from build123d import *

# Parameters (mm, degrees)
CROQUIS1_R              = 12
CROQUIS1_R_2            = 3.25
SALIENTE_EXTRUIR1_DEPTH = 35
SALIENTE_EXTRUIR2_START = -10
CROQUIS2_R              = 12
CROQUIS2_R_2            = 8
SALIENTE_EXTRUIR2_DEPTH = 10
CROQUIS3_R              = 5.1
CROQUIS3_W              = 8
CROQUIS3_H              = 16.86
CORTAR_EXTRUIR2_DEPTH   = 105.669140151


with BuildPart() as part:
    # Croquis1 → Saliente-Extruir1 (new body)
    # profile 1 of 2: a face of its own
    with BuildSketch(Plane.XY):
        with BuildLine():
            Line((0, 85.17), (0, 40.17))
            Line((0, 40.17), (10, 40.17))
            Line((10, 40.17), (10, 60.17))
            Line((10, 60.17), (30, 60.17))
            Line((30, 60.17), (30, 40.17))
            Line((30, 40.17), (40, 40.17))
            Line((40, 40.17), (40, 85.17))
            ThreePointArc((40, 85.17), (38.535533906, 88.705533906), (35, 90.17))
            Line((35, 90.17), (5, 90.17))
            ThreePointArc((5, 90.17), (1.464466094, 88.705533906), (0, 85.17))
        make_face()
        with Locations((20, 74.17)):
            Circle(CROQUIS1_R, mode=Mode.SUBTRACT)
    # profile 2 of 2: a face of its own
    with BuildSketch(Plane.XY):
        with BuildLine():
            Line((5, 0), (35, 0))
            ThreePointArc((35, 0), (38.535533906, 1.464466094), (40, 5))
            Line((40, 5), (40, 40.17))
            Line((40, 40.17), (0, 40.17))
            Line((0, 40.17), (0, 5))
            ThreePointArc((0, 5), (1.464466094, 1.464466094), (5, 0))
        make_face()
        with Locations((20, 4)):
            Circle(CROQUIS1_R_2, mode=Mode.SUBTRACT)
    extrude(amount=SALIENTE_EXTRUIR1_DEPTH)

    # Croquis2 → Saliente-Extruir2 (add)
    with BuildSketch(Plane.XY.offset(35).offset(SALIENTE_EXTRUIR2_START)):
        with Locations((20, 74.17)):
            Circle(CROQUIS2_R)
        with Locations((20, 74.17)):
            Circle(CROQUIS2_R_2, mode=Mode.SUBTRACT)
    extrude(amount=SALIENTE_EXTRUIR2_DEPTH)

    # Croquis3 → Cortar-Extruir2 (cut, through all)
    with BuildSketch(Plane.ZY):
        with Locations((17.5, 27.36)):
            Circle(CROQUIS3_R)
        with Locations((17.5, 8.43)):
            Rectangle(CROQUIS3_W, CROQUIS3_H)
    extrude(amount=-CORTAR_EXTRUIR2_DEPTH, mode=Mode.SUBTRACT)


solid = part.part
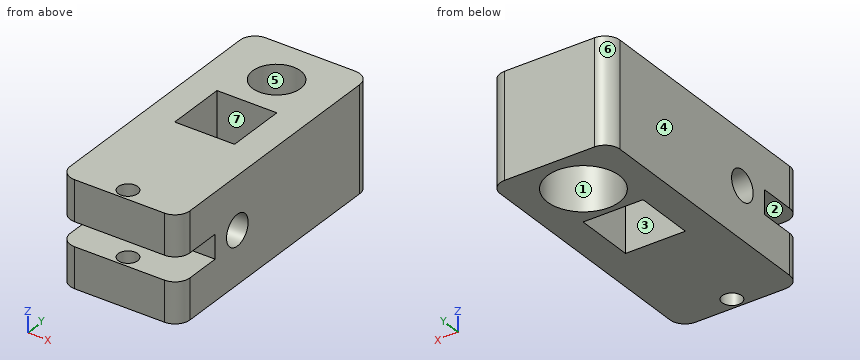
The listing builds one solid part. Answer for the finished solid, in the listing's coordinates (mm). Face numbers are marked on the shaded views. A direction names the side the tool comes from. Coordinates: 2 decimals unless noted, no trailing zeros. Loops run counter-clockwise (first coordinate to the right, second up) from the corner with the lowest first, then second, coordinate; pieces in that order, holes last. Notation, with made-up numbers: (76, 25.5) -> (117, 25.5) arc R29 cw to (117, 58.5) -> close; hole circle Ø9 at (20, 11.25). An arc over 180 degrees is marked (long way). Answer in a Markdown table with one row per item. Add a question column.
1. The part is cut by section C-C, the plane y = 27.36. Write down the section's boundary in (x, z), then the cut area to 3 significant figures.
2. The part is cut by section D-D, the plane z = 31.5. Write down the section's boundary in (x, y), then the cut area to 3 significant figures.
3. The part is cut by section A-A, the plane x = 20. Count the separate pieces of the cut face and the enclosed holes in it, then the cut area to 3 significant figures.
4. Flat-ended cylindrical pins translate along their axes: P1, Ø1.5, axis at x = 27, z = 20, coming from the -Y side; P2, Ø21, axis at x = 20, y = 74.17, coming from the -Z side; P3, Ø4, axis at x = 20, y = 4, coming from the +Z side. Find the tip coordinate at first contact, or state that the pin passes through.
5. For the marked faces 1, 2 and 3, determine the directions among +Z, -Z, +X, -X, +Y, -Y from which every point of the face is accessible in a straight line to the end or side of a thin tool.
6. Consider line 1 (Y direction, x = 20, z = 29); line 2 (X direction, y = 52, z = 9); line 3 (Z direction, x = 30, y = 27). Determine where each line is inside the solid, lowest interval first. Write a range as [from, to].
7. The part is cut by section B-B, the plane z = 17.5. Write down the section's boundary in (x, y), then the cut area to 3 significant figures.
8. Determine the mould class of the marked faces 4, 5, 6 and 7 for opening direction Y: +Y half, -Y half, draft (parallel to the pull), parting line (faces both ways), or undercut.
Answer below:
| question | item | result |
|---|---|---|
| 1 | outline | (0, 0) -> (40, 0) -> (40, 12.4) -> (0, 12.4) -> close; (0, 22.6) -> (40, 22.6) -> (40, 35) -> (0, 35) -> close |
| 1 | area | 992 mm2 |
| 2 | outline | (0, 5) arc R5 ccw to (5, 0) -> (35, 0) arc R5 ccw to (40, 5) -> (40, 85.17) arc R5 ccw to (35, 90.17) -> (5, 90.17) arc R5 ccw to (0, 85.17) -> close; hole (10, 40.17) -> (30, 40.17) -> (30, 60.17) -> (10, 60.17) -> close; hole circle Ø16 at (20, 74.17); hole circle Ø6.5 at (20, 4) |
| 2 | area | 2,950 mm2 |
| 3 | separate pieces | 5 |
| 3 | enclosed holes | 1 |
| 3 | area | 1,300 mm2 |
| 4 | P1 | y = 16.86 |
| 4 | P2 | z = 25 |
| 4 | P3 | through |
| 5 | face 1 | -Z |
| 5 | face 2 | +X, -X, -Y |
| 5 | face 3 | +Z, -Z |
| 6 | line 1 | [0, 0.75], [7.25, 40.17], [60.17, 66.17], [82.17, 90.17] |
| 6 | line 2 | [0, 10], [30, 40] |
| 6 | line 3 | [0, 12.41], [22.59, 35] |
| 7 | outline | (0, 16.86) -> (40, 16.86) -> (40, 22.26) -> (0, 22.26) -> close; (0, 32.46) -> (40, 32.46) -> (40, 85.17) arc R5 ccw to (35, 90.17) -> (5, 90.17) arc R5 ccw to (0, 85.17) -> close; hole circle Ø24 at (20, 74.17); hole (10, 40.17) -> (30, 40.17) -> (30, 60.17) -> (10, 60.17) -> close |
| 7 | area | 1,660 mm2 |
| 8 | face 4 | draft |
| 8 | face 5 | undercut |
| 8 | face 6 | +Y half |
| 8 | face 7 | undercut |
